Can you work these out from the model? Positions are in its coordinate system, mm. A direction names the side the tool comes from. Coordinates: 2 decimals unless noted, no trailing zeros. Order: outer loops, then holes, each group sorted by start corner. A loop starts at its lowest first (then second) coordinate and runs counter-clockwise, first axis right, second up. Notation, with made-up numbers: M -22.5,12 L -11.5,12 A20 ccw -11.5,22 Z; hole C 43,89.25 d3. An arc over 180 degrees is marked long. Answer as a JSON object with one key per item and string values.
from build123d import *

# Parameters (mm, degrees)
SKETCH_1_W          = 44
SKETCH_1_H          = 65
EXTRUDE_1_DEPTH     = 12
CHAMFER_1_SIZE      = 3
CHAMFER_2_SIZE      = 1.5
SKETCH_2_W          = 6
SKETCH_2_H          = 6
SKETCH_2_R          = 1.6
EXTRUDE_2_DEPTH     = 5
FILLET_1_R          = 2
FILLET_2_R          = 2
SKETCH_3_R          = 3
CUT_EXTRUDE_1_DEPTH = 5
SKETCH_4_R          = 2.96404504
EXTRUDE_3_DEPTH     = 5
SKETCH_5_W          = 5.5
SKETCH_5_H          = 6.5
CUT_EXTRUDE_2_DEPTH = 49.53091798


with BuildPart() as part:
    # 草图1 → 凸台-拉伸1 (new body)
    with BuildSketch(Plane(origin=(0, 0, 0), x_dir=(1, 0, 0), z_dir=(0, 1, 0))):
        Rectangle(SKETCH_1_W, SKETCH_1_H)
    extrude(amount=EXTRUDE_1_DEPTH)

    # 倒角1
    chamfer_1_edges = [part.edges().sort_by_distance(p)[0] for p in [
        (22, 6, 32.5),
        (-22, 6, 32.5),
        (-22, 6, -32.5),
        (22, 6, -32.5),
    ]]
    chamfer(chamfer_1_edges, length=CHAMFER_1_SIZE)

    # 倒角2
    chamfer_2_edges = [part.edges().sort_by_distance(p)[0] for p in [
        (-22, 12, 0),
        (0, 12, -32.5),
        (22, 12, 0),
        (0, 12, 32.5),
        (-20.5, 12, 31),
        (20.5, 12, 31),
        (20.5, 12, -31),
        (-20.5, 12, -31),
    ]]
    chamfer(chamfer_2_edges, length=CHAMFER_2_SIZE)

    # 草图2 → 凸台-拉伸2 (add)
    # profile 1 of 2: a face of its own
    with BuildSketch(Plane.XZ):
        with Locations((-6, 35.5)):
            Rectangle(SKETCH_2_W, SKETCH_2_H)
        with Locations(Location((-6, 35.5, 0), (0, 0, 270))):
            Circle(SKETCH_2_R, mode=Mode.SUBTRACT)
    # profile 2 of 2: a face of its own
    with BuildSketch(Plane.XZ):
        with Locations((6, -35.5)):
            Rectangle(SKETCH_2_W, SKETCH_2_H)
        with Locations(Location((6, -35.5, 0), (0, 0, 270))):
            Circle(SKETCH_2_R, mode=Mode.SUBTRACT)
    extrude(amount=-EXTRUDE_2_DEPTH)

    # 圆角1
    fillet_1_edges = [part.edges().sort_by_distance(p)[0] for p in [
        (9, 2.5, -32.5),
        (3, 2.5, -32.5),
        (-3, 2.5, 32.5),
        (-9, 2.5, 32.5),
    ]]
    fillet(fillet_1_edges, radius=FILLET_1_R)

    # 圆角2
    fillet_2_edges = [part.edges().sort_by_distance(p)[0] for p in [
        (9, 2.5, -38.5),
        (3, 2.5, -38.5),
        (-3, 2.5, 38.5),
        (-9, 2.5, 38.5),
    ]]
    fillet(fillet_2_edges, radius=FILLET_2_R)

    # 草图3 → 切除-拉伸1 (cut)
    with BuildSketch(Plane(origin=(22, 0, 0), x_dir=(0, 0, -1), z_dir=(1, 0, 0))):
        with Locations((-20.5, 4.900714175)):
            Circle(SKETCH_3_R)
        with Locations((-10.5, 4.900714175)):
            Circle(SKETCH_3_R)
        with Locations((-0.5, 4.900714175)):
            Circle(SKETCH_3_R)
    extrude(amount=-CUT_EXTRUDE_1_DEPTH, mode=Mode.SUBTRACT)

    # 草图4 → 凸台-拉伸3 (add)
    with BuildSketch(Plane.ZY.offset(22)):
        with Locations(Location((14.738572915, 5.389285653, 0), (0, 0, 180))):
            Circle(SKETCH_4_R)
    extrude(amount=EXTRUDE_3_DEPTH)

    # 草图5 → 切除-拉伸2 (cut, through all)
    with BuildSketch(Plane.XZ):
        with Locations((-13.75, -15.75)):
            Rectangle(SKETCH_5_W, SKETCH_5_H)
    extrude(amount=-CUT_EXTRUDE_2_DEPTH, mode=Mode.SUBTRACT)


solid = part.part
Item 1: I want a section at A-A, the plane z = -35.5. Write out the boundary of the cut face in (x, y).
Answers follow:
{"outline": "M 3,0 L 4.4,0 L 4.4,5 L 3,5 Z; M 7.6,0 L 9,0 L 9,5 L 7.6,5 Z"}
Item 2: I want a section at B-B, the plane x = -6. Write out the boundary of the cut face in (y, z), plus the area to 3 significant figures.
Answers follow:
{"outline": "M 0,-32.5 L 10.5,-32.5 L 12,-31 L 12,31 L 10.5,32.5 L 5,32.5 L 5,33.9 L 0,33.9 Z; M 0,37.1 L 5,37.1 L 5,38.5 L 0,38.5 Z", "area": "792 mm^2"}
Item 3: If we mould it in two halves opening along Z, with no side actions, what happens to faces 6 (the flat face through (-21.2, 11.3, 0.4)), 7 (the flat face through (0, 5, -32.5)), 8 (the flat face through (17, 5, 1))? For each: pulls with the +Z half, pulls with the -Z half, needs draft (parallel to the pull), parting line crosses it, or undercut.
Answers follow:
{"face 6": "needs draft", "face 7": "pulls with the -Z half", "face 8": "undercut"}
Item 4: I want a section at C-C, the plane y = 9.75. Write out the boundary of the cut face in (x, z), plus the area to 3 significant figures.
Answers follow:
{"outline": "M -22,-29.5 L -19,-32.5 L 19,-32.5 L 22,-29.5 L 22,29.5 L 19,32.5 L -19,32.5 L -22,29.5 Z; hole M -16.5,-19 L -11,-19 L -11,-12.5 L -16.5,-12.5 Z", "area": "2,810 mm^2"}
Item 5: I'm going to push flat-ended pins straight in: pin 1 (5.5 mm diameter, centred on y = 4.9, z = 10.5, fed in from +X); pin 2 (6.5 mm diameter, centred on x = 7, z = -34.5, fed in from +Y); pin 3 (0.6 mm diameter, centred on y = 2.5, z = 36, fed in from -X). Where does each tip first touch, or does it pass through?
Answers follow:
{"pin 1": "stops at x = 17", "pin 2": "stops at y = 11.75", "pin 3": "stops at x = -9"}
Item 6: Please list where these lines run through material, in increasing order: line 1 (X direction, y = 3.7, z = 35.5); line 2 (Z direction, x = 13.5, y = 3.5); line 3 (X direction, y = 8.5, z = 5.5).
Answers follow:
{"line 1": "x = -9 to -7.6, -4.4 to -3", "line 2": "z = -32.5 to 32.5", "line 3": "x = -22 to 22"}
Item 7: Which directions (+Z, -Z, +X, -X, +Y, -Y) give clear straight access to the entire face, cutting with the end or side of a thin tool? Please do faces 1 (the flat face through (-14, 6, -12.5)), 2 (the flat face through (-6, 2, 38.5)), 3 (the cylindrical face through (-2.4, 2.54, 33.07)), 4 (the flat face through (-9, 2, 35)), 5 (the flat face through (7, 5, -34)).
Answers follow:
{"face 1": "+Y, -Y", "face 2": "+Z, +X, -X, +Y, -Y", "face 3": "+Z, +X, +Y, -Y", "face 4": "+Z, -X, +Y, -Y", "face 5": "-Z, +X, -X, +Y"}
Item 8: I want a section at D-D, the plane z = 10.5. Write out the boundary of the cut face in (x, y), plus the area to 3 significant figures.
Answers follow:
{"outline": "M -22,0 L 22,0 L 22,1.9 L 17,1.9 L 17,7.9 L 22,7.9 L 22,10.5 L 20.5,12 L -20.5,12 L -22,10.5 Z", "area": "496 mm^2"}
